For this review, take the finished solid that the model builds, in its own axes (mm). A direction names the side the tool comes from. Give positions to 0.01 mm unless a question says otherwise; leave off trailing zeros. Write each loop counter-clockwise with the first axis right and the second up, starting at its lowest first coordinate (ties: lowest second). Pieces come first, ordered by that corner, then holes.
1) We need section D-D on x = 19.5. Give the boundary of the cut face in (y, z).
2) We need section A-A on y = 0. Give the boundary of the cut face in (x, z).
3) Wall thickness on line 1 along Y through (x, z) = (19.5, 14.5); line 2 along Y through (x, z) = (0, 16); line 3 along Y through (x, z) = (0, 7.75): over which ranges is each line inside the solid? List them lowest first.
4) Machinability: for faces 4 (the face through (-9.2, 15.1, 22)), 5 (the face through (-0.46, 17.2, 7.95)), 6 (the face through (20.013, -4.444, 21.014)), which of the approach directions +Z, -Z, +X, -X, +Y, -Y give a long, thin tool a straight path to every point of the face, cutting with its end or side? Answer none if there is none.
5) We need section C-C on x = -4. Give the boundary of the cut face in (y, z), and give its area (3 significant figures).
6) For P1, Ø1.5, axis at y = -11, z = 23, coming from the +X side; P2, Ø3.5, axis at x = 0, z = 10, coming from the +Y side; P3, Ø5, axis at x = 19.5, y = -19.5, coming from the +Z side; P4, Ø1, axis at x = 6, y = -11.5, coming from the -Z side, all flat-tipped, find the tip position at first contact; note any pin that passes through.
7) Draft analysis for pull direction X (two halves, no side actions). For faces 1 (the face through (-22, 0, 20)), 2 (the face through (24.5, 0, 10)), 3 (the face through (-6.466, -2.681, 13.804)), state which applies: pulls with the +X half, pulls with the -X half, needs draft (parallel to the pull), parting line crosses it, or undercut.
8) We need section B-B on z = 14.5. Give the boundary of the cut face in (x, y), and give its area (3 significant figures).
from build123d import *

# Parameters (mm, degrees)
F0_W     = 49
F0_H     = 49
F1_DEPTH = 20
F3_D     = 6
F7_D     = 4.2
F7_DEPTH = 14.4
F7_TIP   = 1.2618073
F9_D     = 4
F9_DEPTH = 18
F9_TIP   = 1.2017212381
F11_D    = 14


with BuildPart() as f1:
    # F0 (on Top) → F1 (new body)
    with BuildSketch(Plane.XY):
        Rectangle(F0_W, F0_H)
    extrude(amount=F1_DEPTH)

    # F3 (through all)
    with Locations(Plane.XY.offset(20)):
        with Locations((-19.5, -19.5), (-19.5, 19.5), (19.5, 19.5), (19.5, -19.5)):
            Hole(F3_D / 2)

    # F4 (on Right) → F5 (revolve)
    with BuildSketch(Plane.YZ):
        Polygon((0, 28), (0, 20), (20.5, 20), (20.5, 22), (17.5, 22), (17.5, 26), (20.5, 26), (20.5, 28), align=None)
    revolve(axis=Axis((0, 0, 24), (0, 0, 1)))

    # F7
    with Locations(Plane(origin=(0, 24.5, 0), x_dir=(-1, 0, 0), z_dir=(0, 1, 0))):
        with Locations((0, 10)):
            Hole(F7_D / 2, depth=F7_DEPTH)
            with Locations((0, 0, -(F7_DEPTH + F7_TIP / 2))):  # 118° drill point
                Cone(0, F7_D / 2, F7_TIP, mode=Mode.SUBTRACT)

    # F9
    with Locations(Plane.XY.offset(28)):
        with Locations((0, 12.5)):
            Hole(F9_D / 2, depth=F9_DEPTH)
            with Locations((0, 0, -(F9_DEPTH + F9_TIP / 2))):  # 118° drill point
                Cone(0, F9_D / 2, F9_TIP, mode=Mode.SUBTRACT)

    # F11 (through all)
    with Locations(Plane.XY.offset(28)):
        with Locations((0, 0)):
            Hole(F11_D / 2)


solid = f1.part
Results list:
1. outline: (-24.5, 0) - (-22.5, 0) - (-22.5, 20) - (-24.5, 20) - close; (-16.5, 0) - (16.5, 0) - (16.5, 20) - (6.32, 20) - (6.32, 22) - (-6.32, 22) - (-6.32, 20) - (-16.5, 20) - close; (-6.32, 26) - (6.32, 26) - (6.32, 28) - (-6.32, 28) - close; (22.5, 0) - (24.5, 0) - (24.5, 20) - (22.5, 20) - close
2. outline: (-24.5, 0) - (-7, 0) - (-7, 28) - (-20.5, 28) - (-20.5, 26) - (-17.5, 26) - (-17.5, 22) - (-20.5, 22) - (-20.5, 20) - (-24.5, 20) - close; (7, 0) - (24.5, 0) - (24.5, 20) - (20.5, 20) - (20.5, 22) - (17.5, 22) - (17.5, 26) - (20.5, 26) - (20.5, 28) - (7, 28) - close
3. line 1: y = -24.5 to -22.5, -16.5 to 16.5, 22.5 to 24.5
3. line 2: y = -24.5 to -7, 7 to 10.5, 14.5 to 24.5
3. line 3: y = -24.5 to -7, 7 to 24.5
4. face 4: none
4. face 5: +Y
4. face 6: +Z
5. outline: (-24.5, 0) - (-5.74, 0) - (-5.74, 28) - (-20.11, 28) - (-20.11, 26) - (-17.04, 26) - (-17.04, 22) - (-20.11, 22) - (-20.11, 20) - (-24.5, 20) - close; (5.74, 0) - (24.5, 0) - (24.5, 20) - (20.11, 20) - (20.11, 22) - (17.04, 22) - (17.04, 26) - (20.11, 26) - (20.11, 28) - (5.74, 28) - close
5. area: 955 mm2
6. P1: stops at x = 14.18
6. P2: stops at y = 9.89
6. P3: passes through
6. P4: stops at z = 0
7. face 1: needs draft
7. face 2: pulls with the +X half
7. face 3: undercut
8. outline: (-24.5, -24.5) - (24.5, -24.5) - (24.5, 24.5) - (-24.5, 24.5) - close; hole circle Ø6 at (-19.5, -19.5); hole circle Ø6 at (-19.5, 19.5); hole circle Ø14 at (0, 0); hole circle Ø4 at (0, 12.5); hole circle Ø6 at (19.5, -19.5); hole circle Ø6 at (19.5, 19.5)
8. area: 2,120 mm2
